from build123d import *

# Parameters (mm, degrees)
SKETCH_W     = 60
SKETCH_H     = 30
PAD_DEPTH    = 5
SKETCH001_W  = 52
SKETCH001_H  = 22
POCKET_DEPTH = 3


with BuildPart() as part:
    # Sketch → Pad (new body)
    with BuildSketch(Plane.XY):
        Rectangle(SKETCH_W, SKETCH_H)
    extrude(amount=PAD_DEPTH)

    # Sketch001 (on DatumPlane) → Pocket (cut)
    with BuildSketch(Plane.XY.offset(5)):
        Rectangle(SKETCH001_W, SKETCH001_H)
    extrude(amount=-POCKET_DEPTH, mode=Mode.SUBTRACT)


solid = part.part
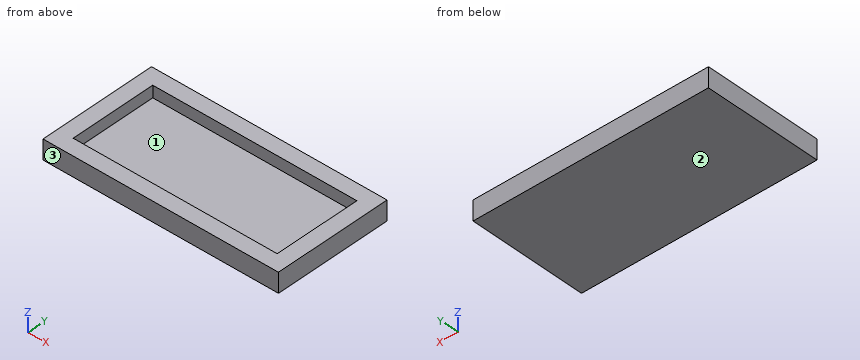
Model file for the job. Use its own axes, mm. Face numbers are marked on the shaded views. Round coordinates to 2 decimals unless told otherwise and drop trailing zeros. Loops run counter-clockwise (first coordinate to the right, second up) from the corner with the lowest first, then second, coordinate; pieces in that order, holes last. Notation, with made-up numbers: (27.5, 79) -> (59.5, 79) arc R19 ccw to (59.5, 95) -> close; hole circle Ø1 at (4, 43.5). An arc over 180 degrees is marked (long way). Answer as CSV lines item,"result". Start each with the question number.
1) Slice it at C-C (x = -8). List the corners of the cut face in (y, z), plus the area to 3 significant figures.
2) Pin check, flat tip, straight feed: P1, Ø11, axis at x = 12, y = 2.5, coming from the +Z side. Stop position of the tip, or through.
3) Slice it at B-B (y = -8). List the corners of the cut face in (x, z), plus the area to 3 significant figures.
4) Mould opens along Y. For the marked faces 1, 2 and 3 say: +Y half, -Y half, draft (parallel to the pull), parting line (faces both ways), or undercut.
5) Probe line 1 along X through (y, z) = (2.75, 3.6); line 2 along Y through (x, z) = (12, 2.55); line 3 along Z through (x, y) = (3.5, -4.75). List the from-to ranges inside material, lowest first.
6) Slice it at A-A (z = 4.4). List the corners of the cut face in (x, y).
Filled in:
1,outline,"(-15, 0) -> (15, 0) -> (15, 5) -> (11, 5) -> (11, 2) -> (-11, 2) -> (-11, 5) -> (-15, 5) -> close"
1,area,"84.0 mm2"
2,P1,"stops at z = 2"
3,outline,"(-30, 0) -> (30, 0) -> (30, 5) -> (26, 5) -> (26, 2) -> (-26, 2) -> (-26, 5) -> (-30, 5) -> close"
3,area,"144 mm2"
4,face 1,"undercut"
4,face 2,"draft"
4,face 3,"-Y half"
5,line 1,"x = -30 to -26, 26 to 30"
5,line 2,"y = -15 to -11, 11 to 15"
5,line 3,"z = 0 to 2"
6,outline,"(-30, -15) -> (30, -15) -> (30, 15) -> (-30, 15) -> close; hole (-26, -11) -> (26, -11) -> (26, 11) -> (-26, 11) -> close"
